Check sheet for the modelled part. Datum: model origin and axes. Units: mm. Face numbers are marked on the shaded views. A direction names the side the tool comes from. Coordinates: 2 decimals unless noted, no trailing zeros. Write each loop counter-clockwise with the first axis right and the second up, starting at its lowest first coordinate (ties: lowest second). Pieces come first, ordered by that corner, then holes. Notation, with made-up numbers: (-24, 11) -> (-20, 11) arc R7 ccw to (-20, 20) -> close; hole circle Ø1 at (73, -17.5). An arc over 180 degrees is marked (long way). One line per item, written item: value. Start each with the question number.
1) Sectioned sample at B-B on x = 19.61. Enter the section's corners in (y, z), plus the area to 3 significant figures.
2) Sectioned sample at D-D on y = 27.32. Enter the section's corners in (x, z).
3) Scan lines: line 1 along Z through (x, y) = (19.61, 0.8); line 2 along Z through (x, y) = (1, 27); line 3 along X through (y, z) = (4, -11.5). Record each from-to range of solid material in increasing order. Write a range as [from, to].
4) Sectioned sample at A-A on y = 10. Enter the section's corners in (x, z), plus the area to 3 significant figures.
5) Gauge pin test, flat ends, axial feed: P1, Ø3, axis at x = 29.5, z = 9.5, coming from the +Y side; P2, Ø3, axis at x = 19.61, z = 0, coming from the -Y side; P3, Ø6, axis at y = 10, z = -5, coming from the +X side. Record the tip position at first contact, or that the pin passes through.
6) Set-up check for the marked faces 1 and 2: record each of +Z, -Z, +X, -X, +Y, -Y from which the full face is reachable in a straight line by a thin tool's end or side.
7) Sectioned sample at C-C on y = 15. Enter the section's corners in (x, z), plus the area to 3 significant figures.
```python
from build123d import *

# Parameters (mm, degrees)
BOSS_EXTRUDE1_DEPTH   = 15
F_6_CLEARANCE_HOLE1_D = 3.7973
FILLET1_R             = 10
F_6_CLEARANCE_HOLE2_D = 3.7973


with BuildPart() as part:
    # Sketch2 → Boss-Extrude1 (new, symmetric)
    with BuildSketch(Plane.XY):
        Polygon((0, 0), (50, 0), (50, 1.5875), (1.5875, 1.5875), (1.5875, 32.32), (0, 32.32), align=None)
    extrude(amount=BOSS_EXTRUDE1_DEPTH, both=True)

    # #6 Clearance Hole1 (through all)
    with Locations(Plane.ZY):
        with Locations((-5, 27.32), (5, 10), (5, 27.32), (-5, 10)):
            Hole(F_6_CLEARANCE_HOLE1_D / 2)

    # Fillet1
    fillet1_edges = [part.edges().sort_by_distance(p)[0] for p in [
        (50, 0.79375, 15),
        (0.79375, 32.32, 15),
        (0.79375, 32.32, -15),
        (50, 0.79375, -15),
    ]]
    fillet(fillet1_edges, radius=FILLET1_R)

    # #6 Clearance Hole2 (through all)
    with Locations(Plane(origin=(0, 0, 0), x_dir=(-1, 0, 0), z_dir=(0, -1, 0))):
        with Locations((-19.61, 0), (-39.61, 0)):
            Hole(F_6_CLEARANCE_HOLE2_D / 2)


solid = part.part
```
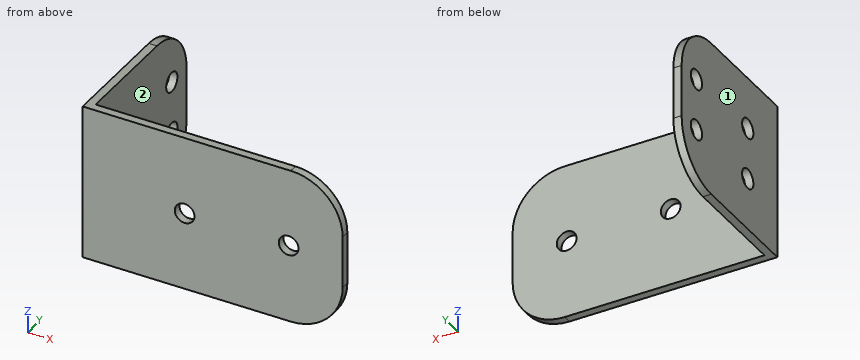
Answers:
1. outline: (0, -15) -> (1.59, -15) -> (1.59, -1.9) -> (0, -1.9) -> close; (0, 1.9) -> (1.59, 1.9) -> (1.59, 15) -> (0, 15) -> close
1. area: 41.6 mm2
2. outline: (0, -13.66) -> (1.59, -13.66) -> (1.59, -6.9) -> (0, -6.9) -> close; (0, -3.1) -> (1.59, -3.1) -> (1.59, 3.1) -> (0, 3.1) -> close; (0, 6.9) -> (1.59, 6.9) -> (1.59, 13.66) -> (0, 13.66) -> close
3. line 1: z = [-15, -1.9], [1.9, 15]
3. line 2: z = [-13.84, -6.87], [-3.13, 3.13], [6.87, 13.84]
3. line 3: x = [0, 1.59]
4. outline: (0, -15) -> (1.59, -15) -> (1.59, -6.9) -> (0, -6.9) -> close; (0, -3.1) -> (1.59, -3.1) -> (1.59, 3.1) -> (0, 3.1) -> close; (0, 6.9) -> (1.59, 6.9) -> (1.59, 15) -> (0, 15) -> close
4. area: 35.6 mm2
5. P1: stops at y = 1.59
5. P2: passes through
5. P3: stops at x = 1.59
6. face 1: +Z, -Z, -X, +Y, -Y
6. face 2: +Z, -Z, +X, +Y
7. outline: (0, -15) -> (1.59, -15) -> (1.59, 15) -> (0, 15) -> close
7. area: 47.6 mm2
